Build history of the part. All positions in model axes, mm. Face numbers are marked on the shaded views. A direction names the side the tool comes from. Give positions to 0.01 mm unless a question says otherwise; leave off trailing zeros. Write each loop counter-clockwise with the first axis right and the second up, starting at its lowest first coordinate (ties: lowest second). Pieces come first, ordered by that corner, then holes. Notation, with made-up numbers: (3.25, 26.25) -> (59.25, 26.25) arc R20 ccw to (59.25, 60.25) -> close; hole circle Ø4 at (79, 31.25). An arc over 180 degrees is marked (long way). Put each result on its own line as item: value. Start each with the question number.
Item 1: Slice it at A-A, the plane z = 8.5. List the corners of the cut face in (x, y).
Item 2: Drill centre lines: line 1 along Z through (x, y) = (3.5, 1.5); line 2 along Y through (x, z) = (11.5, 2); line 3 along Y through (x, z) = (14, 10.75). Where is each one in solid material? Low to high.
Item 3: Two-plate mould, pull along X, no slides. Class the marked faces 1, 2, 3 and 4: pulls with the +X half, pulls with the -X half, needs draft (parallel to the pull), parting line crosses it, or undercut.
Item 4: Tool access for the marked faces 5 and 6: list every direction of +Z, -Z, +X, -X, +Y, -Y with a clear straight run to the whole face (end or side of a thin tool).
Item 5: Slice it at B-B, the plane y = 0. List the corners of the cut face in (x, z).
Item 6: Slice it at C-C, the plane x = -11. List the corners of the cut face in (y, z).
Item 7: Flat gauge pins, fed straight in: pin 1 Ø6 at (x, z) = (11.5, 4) entering from +Y; pin 2 Ø1.5 at (x, y) = (7.5, 9.5) entering from +Z; pin 3 Ø4 at (x, z) = (8, 8) entering from +Y (3 decimals); pin 4 Ø5 at (x, z) = (10.5, 7) entering from +Y. Where does each tip first touch, or does it go through?
Item 8: Slice it at D-D, the plane z = 0.5. List the corners of the cut face in (x, y) (3 decimals).
```python
from build123d import *

# Parameters (mm, degrees)
F0_R            = 21.5
F0_R_2          = 13.5
F1_DEPTH        = 5
F3_DEPTH        = 6
F4_R            = 5.125
F5_DEPTH        = 4.5
F7_END_RADIUS   = 13.5
F7_REACH        = 39.2960714607
F7_COPIES_COUNT = 7


# Not quite as in the source:
# - a pattern or mirror of a feature is missing from the dataset's text; its kind, count and spacing are read off the source's solid


with BuildPart() as f1:
    # F0 (on Top) → F1 (new body)
    with BuildSketch(Plane.XY):
        Circle(F0_R)
        Circle(F0_R_2, mode=Mode.SUBTRACT)
        Circle(F0_R_2)
    extrude(amount=F1_DEPTH)

    # F2 (on face) → F3 (join)
    with BuildSketch(Plane.XY.offset(5)):
        with BuildLine():
            ThreePointArc((-13.4614857204, -1.0190202158), (-13.5, 0), (-13.4614857204, 1.0190202158))
            Line((-13.4614857204, 1.0190202158), (-15.4614857204, 1.0190202158))
            Line((-15.4614857204, 1.0190202158), (-15.4614857204, -1.0190202158))
            Line((-15.4614857204, -1.0190202158), (-13.4614857204, -1.0190202158))
        make_face()
        with BuildLine():
            ThreePointArc((-7.5963969786, -11.1599620494), (-8.4171123251, -10.5547250133), (-9.1898011505, -9.8892646246))
            Line((-9.1898011505, -9.8892646246), (-10.4367807542, -11.4529275895))
            Line((-10.4367807542, -11.4529275895), (-8.8433765823, -12.7236250143))
            Line((-8.8433765823, -12.7236250143), (-7.5963969786, -11.1599620494))
        make_face()
        with BuildLine():
            ThreePointArc((3.9889336264, -12.8972248381), (3.0040326084, -13.1615268145), (2.0019911235, -13.3507314984))
            Line((2.0019911235, -13.3507314984), (2.4470329914, -15.3005873227))
            Line((2.4470329914, -15.3005873227), (4.4339754943, -14.8470806625))
            Line((4.4339754943, -14.8470806625), (3.9889336264, -12.8972248381))
        make_face()
        with BuildLine():
            ThreePointArc((12.5705158512, -4.9226142683), (12.1630797167, -5.8574304781), (11.6862432483, -6.7588252486))
            Line((11.6862432483, -6.7588252486), (13.4881809841, -7.6265927268))
            Line((13.4881809841, -7.6265927268), (14.372453587, -5.7903817465))
            Line((14.372453587, -5.7903817465), (12.5705158512, -4.9226142683))
        make_face()
        with BuildLine():
            ThreePointArc((11.6862432483, 6.7588252486), (12.1630797167, 5.8574304781), (12.5705158512, 4.9226142683))
            Line((12.5705158512, 4.9226142683), (14.372453587, 5.7903817465))
            Line((14.372453587, 5.7903817465), (13.4881809841, 7.6265927268))
            Line((13.4881809841, 7.6265927268), (11.6862432483, 6.7588252486))
        make_face()
        with BuildLine():
            ThreePointArc((2.0019911235, 13.3507314984), (3.0040326084, 13.1615268145), (3.9889336264, 12.8972248381))
            Line((3.9889336264, 12.8972248381), (4.4339754943, 14.8470806625))
            Line((4.4339754943, 14.8470806625), (2.4470329914, 15.3005873227))
            Line((2.4470329914, 15.3005873227), (2.0019911235, 13.3507314984))
        make_face()
        with BuildLine():
            ThreePointArc((-9.1898011505, 9.8892646246), (-8.4171123251, 10.5547250133), (-7.5963969786, 11.1599620494))
            Line((-7.5963969786, 11.1599620494), (-8.8433765823, 12.7236250143))
            Line((-8.8433765823, 12.7236250143), (-10.4367807542, 11.4529275895))
            Line((-10.4367807542, 11.4529275895), (-9.1898011505, 9.8892646246))
        make_face()
    extrude(amount=F3_DEPTH)

    # F4 (on face) → F5 (cut)
    with BuildSketch(Plane(origin=(0, 0, 0), x_dir=(1, 0, 0), z_dir=(0, 0, -1))):
        with Locations((-14.875, 0)):
            Circle(F4_R)
        with Locations((14.875, 0)):
            Circle(F4_R)
    extrude(amount=-F5_DEPTH, mode=Mode.SUBTRACT)

    f7_end = (Plane(origin=(0, 0, 8), x_dir=(-1, 0, 0), z_dir=(0, 0, -1)) * Cylinder(F7_END_RADIUS, 202.1882593652, mode=Mode.PRIVATE)).faces().sort_by_distance((-13.5, 0, 8))[0]
    # F6 (on face) → F7 (join, up to the whole of a round face its end follows)
    with BuildSketch(Plane(origin=(-15.4614857204, 0, 0), x_dir=(0, -1, 0), z_dir=(-1, 0, 0))):
        Polygon((1.0190202158, 6.5), (1.0190202158, 5), (2.8066506047, 6.5), align=None)
    f7_long = extrude(amount=-F7_REACH, mode=Mode.PRIVATE)
    f7 = split(f7_long, bisect_by=f7_end, keep=Keep.ALL, mode=Mode.PRIVATE).solids().sort_by_distance((-15.4614857204, -1.6148970121, 6))[0]
    add(f7)

    # F7_copies: F7 ×7 about axis
    f7_copies_axis = Axis((0, 0, 0), (0, 0, 1))
    for i in range(1, F7_COPIES_COUNT):
        add(f7.rotate(f7_copies_axis, i * 360 / F7_COPIES_COUNT))


solid = f1.part
```
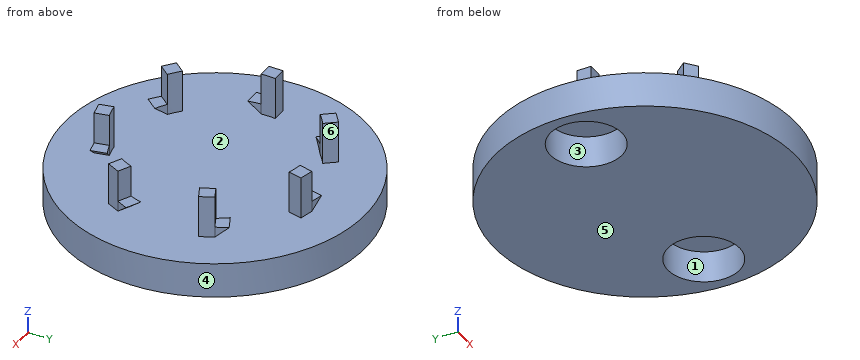
Values follow:
1. outline: (-15.46, -1.02) -> (-13.46, -1.02) arc R13.5 cw to (-13.46, 1.02) -> (-15.46, 1.02) -> close; (-10.44, -11.45) -> (-8.84, -12.72) -> (-7.6, -11.16) arc R13.5 cw to (-9.19, -9.89) -> close; (-10.44, 11.45) -> (-9.19, 9.89) arc R13.5 cw to (-7.6, 11.16) -> (-8.84, 12.72) -> close; (2, -13.35) -> (2.45, -15.3) -> (4.43, -14.85) -> (3.99, -12.9) arc R13.5 cw to start; (2, 13.35) arc R13.5 cw to (3.99, 12.9) -> (4.43, 14.85) -> (2.45, 15.3) -> close; (11.69, -6.76) -> (13.49, -7.63) -> (14.37, -5.79) -> (12.57, -4.92) arc R13.5 cw to start; (11.69, 6.76) arc R13.5 cw to (12.57, 4.92) -> (14.37, 5.79) -> (13.49, 7.63) -> close
2. line 1: 0 to 5
2. line 2: -18.17 to -3.86, 3.86 to 18.17
2. line 3: -6.56 to -5.61, 5.61 to 6.56
3. face 1: undercut
3. face 2: needs draft
3. face 3: undercut
3. face 4: parting line crosses it
4. face 5: -Z, +X, -X, +Y, -Y
4. face 6: +Z, +X, +Y
5. outline: (-21.5, 0) -> (-20, 0) -> (-20, 4.5) -> (-9.75, 4.5) -> (-9.75, 0) -> (9.75, 0) -> (9.75, 4.5) -> (20, 4.5) -> (20, 0) -> (21.5, 0) -> (21.5, 5) -> (-13.5, 5) -> (-13.5, 11) -> (-15.46, 11) -> (-15.46, 5) -> (-21.5, 5) -> close
6. outline: (-18.47, 0) -> (-3.35, 0) -> (-3.35, 4.5) -> (3.35, 4.5) -> (3.35, 0) -> (18.47, 0) -> (18.47, 5) -> (-18.47, 5) -> close; (9.29, 6.5) -> (11, 5.6) -> (11, 6.5) -> close
7. pin 1: y = 19.75
7. pin 2: z = 5
7. pin 3: through
7. pin 4: y = 19.53
8. outline: circle Ø43 at (0, 0); hole circle Ø10.25 at (-14.875, 0); hole circle Ø10.25 at (14.875, 0)
